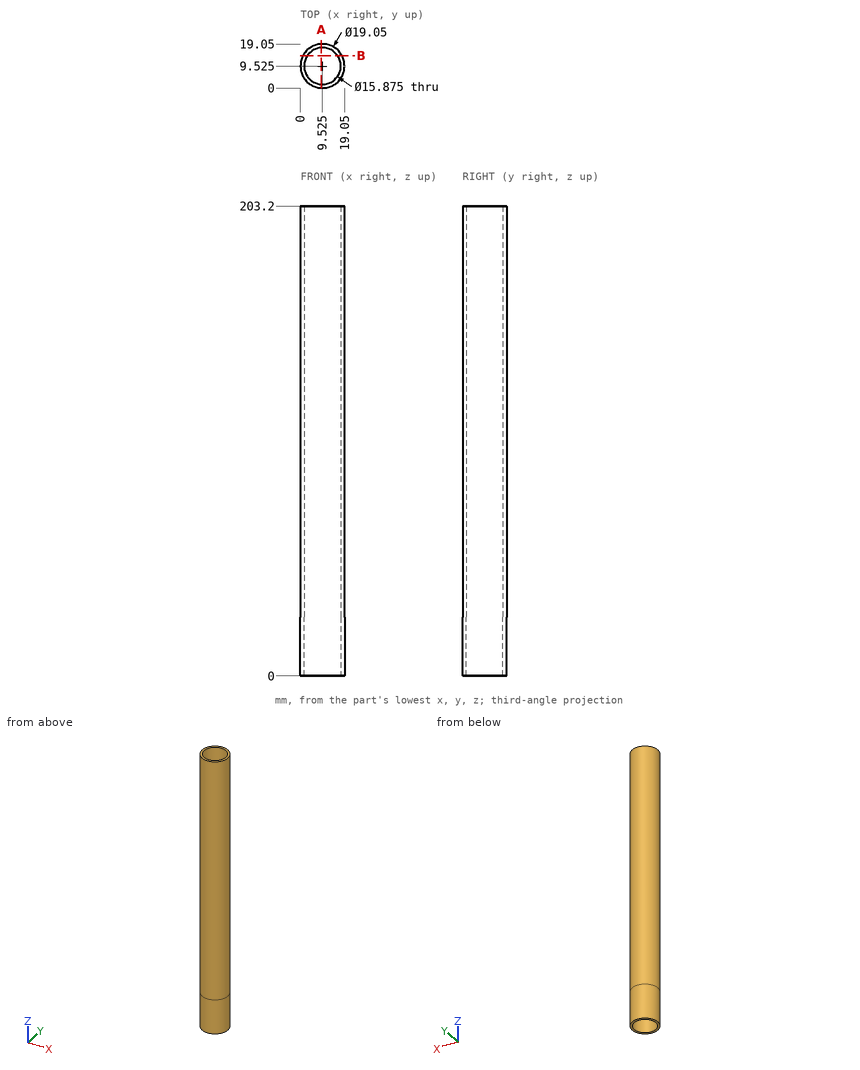
Input: dimensioned drawing with shaded views. Units: mm. Origin: part minimum x, y, z. Round coordinates to 2 decimals unless told otherwise and drop trailing zeros. Order: outer loops, then holes, each group sorted by start corner. A loop starts at its lowest first (then second) coordinate and runs counter-clockwise, first axis right, second up. Notation, with made-up numbers: (45, 22.25) -> (85, 22.25) arc R23 cw to (85, 61.25) -> close; hole circle Ø2 at (54.5, -28). An arc over 180 degrees is marked (long way). One line per item, written item: value. Start each with the question number.
Q1. Material intervals for probe 1 along Y at (x, z) = (9.5, 163.5); probe 2 along Y at (x, z) = (9, 83), sorted ascending.
Q2. Pin query (flat end, axial travel): pin 1 (5 mm diameter, centred on y = 6.5, z = 67, fed in from +X); pin 2 (1.5 mm diameter, centred on y = 7, z = 70.5, fed in from -X); pin 3 (4 mm diameter, centred on y = 3.5, z = 81, fed in from +X). Return the tip coordinate at first contact, or that it passes through.
Q3. Section query B-B (y = 14). Return the cut outline in (x, z), plus the area to 3 significant figures.
Q4. Section query A-A (x = 9). Return the cut outline in (y, z), plus the area to 3 significant figures.
Findings below:
1. probe 1: 0 to 1.59, 17.46 to 19.05
1. probe 2: 0.01 to 1.6, 17.45 to 19.04
2. pin 1: x = 19.04
2. pin 2: x = 0.17
2. pin 3: x = 18.16
3. outline: (1.12, 0) -> (2.97, 0) -> (2.97, 203.2) -> (1.12, 203.2) -> close; (16.08, 0) -> (17.93, 0) -> (17.93, 203.2) -> (16.08, 203.2) -> close
3. area: 753 mm²
4. outline: (0.01, 0) -> (1.6, 0) -> (1.6, 203.2) -> (0.01, 203.2) -> close; (17.45, 0) -> (19.04, 0) -> (19.04, 203.2) -> (17.45, 203.2) -> close
4. area: 646 mm²
